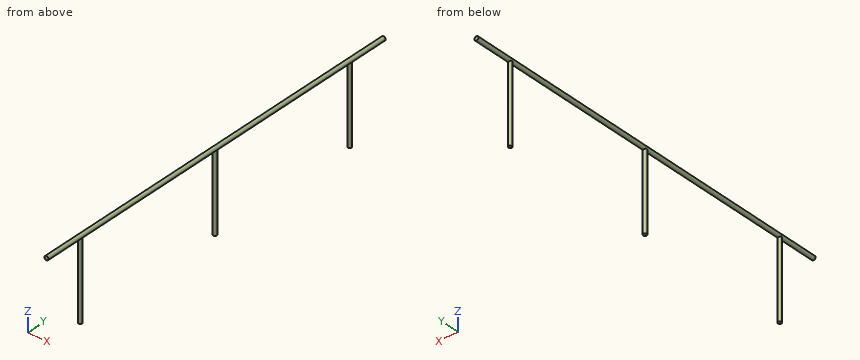
from build123d import *

# Parameters (mm, degrees)
F0_R     = 12.7
F1_DEPTH = 1250
F2_R     = 11.2
F3_DEPTH = 500


with BuildPart() as f1:
    # F0 (on Front) → F1 (new body, symmetric)
    with BuildSketch(Plane.XZ):
        Circle(F0_R)
    extrude(amount=F1_DEPTH, both=True)

    # F2 (on Top) → F3 (join)
    with BuildSketch(Plane.XY):
        Circle(F2_R)
        with Locations((0, -1000)):
            Circle(F2_R)
        with Locations((0, 1000)):
            Circle(F2_R)
    extrude(amount=-F3_DEPTH)


solid = f1.part
Geometry check sheet. Reference: the model listing, model coordinates, mm. Give positions to 0.01 mm unless a question says otherwise; leave off trailing zeros. Write each loop counter-clockwise with the first axis right and the second up, starting at its lowest first coordinate (ties: lowest second). Pieces come first, ordered by that corner, then holes. Notation, with made-up numbers: M -20.75,45 L 10.25,45 A12 ccw 10.25,53 Z; hole C -8,9 d7. An arc over 180 degrees is marked long. One line per question, with ' | ' between items.
1. Cross-section at A-A (z = -464). Enter the section's corners in (x, y).
Ans:
outline: C 0,-1000 d22.4; C 0,0 d22.4; C 0,1000 d22.4
2. Scan lines: line 1 along Y through (x, z) = (-2, -421); line 2 along Y through (x, z) = (-2.5, -128.5); line 3 along Z through (x, y) = (-1, 441). Record each from-to range of solid material in increasing order. Write a range as from..to.
Ans:
line 1: -1011.02..-988.98, -11.02..11.02, 988.98..1011.02 | line 2: -1010.92..-989.08, -10.92..10.92, 989.08..1010.92 | line 3: -12.66..12.66
3. Cross-section at C-C (y = -74.5). Enter the section's corners in (x, z).
Ans:
outline: C 0,0 d25.4
4. Cross-section at B-B (x = -6.25). Enter the section's corners in (y, z), plus the area to 3 significant figures.
Ans:
outline: M -1250,-11.06 L -1009.29,-11.06 L -1009.29,-500 L -990.71,-500 L -990.71,-11.06 L -9.29,-11.06 L -9.29,-500 L 9.29,-500 L 9.29,-11.06 L 990.71,-11.06 L 990.71,-500 L 1009.29,-500 L 1009.29,-11.06 L 1250,-11.06 L 1250,11.06 L -1250,11.06 Z | area: 82,500 mm2
5. Gauge pin test, flat ends, axial feed: pin 1 (3 mm diameter, centred on x = 8, y = -266, fed in from +Z); pin 2 (1.5 mm diameter, centred on x = -9.5, z = -116.5, fed in from -Y); pin 3 (1.5 mm diameter, centred on x = 1.5, y = 638.5, fed in from +Z). Record the tip position at first contact, or that the pin passes through.
Ans:
pin 1: z = 10.91 | pin 2: y = -1006.99 | pin 3: z = 12.68
